```python
from build123d import *

# Parameters (mm, degrees)
SKETCH_R   = 95
SKETCH_R_2 = 7
SKETCH_R_3 = 1.5
SKETCH_R_4 = 2.5
PAD_DEPTH  = 4


with BuildPart() as part:
    # Sketch → Pad (new body)
    with BuildSketch(Plane.XY):
        Circle(SKETCH_R)
        with Locations((-45, 0)):
            Circle(SKETCH_R_2, mode=Mode.SUBTRACT)
        with Locations((45, 0)):
            Circle(SKETCH_R_2, mode=Mode.SUBTRACT)
        with Locations((64.346717, 64.346717)):
            Circle(SKETCH_R_3, mode=Mode.SUBTRACT)
        with Locations((-64.346717, 64.346717)):
            Circle(SKETCH_R_3, mode=Mode.SUBTRACT)
        with Locations((-64.346717, -64.346717)):
            Circle(SKETCH_R_3, mode=Mode.SUBTRACT)
        with Locations((64.346717, -64.346717)):
            Circle(SKETCH_R_3, mode=Mode.SUBTRACT)
        with Locations((-45, 19.5)):
            Circle(SKETCH_R_4, mode=Mode.SUBTRACT)
        with Locations((-28.112505, -9.75)):
            Circle(SKETCH_R_4, mode=Mode.SUBTRACT)
        with Locations((-61.887495, -9.75)):
            Circle(SKETCH_R_4, mode=Mode.SUBTRACT)
        with Locations((45, 19.5)):
            Circle(SKETCH_R_4, mode=Mode.SUBTRACT)
        with Locations((28.112505, -9.75)):
            Circle(SKETCH_R_4, mode=Mode.SUBTRACT)
        with Locations((61.887495, -9.75)):
            Circle(SKETCH_R_4, mode=Mode.SUBTRACT)
        Circle(SKETCH_R_4, mode=Mode.SUBTRACT)
        with Locations((91, 0)):
            Circle(SKETCH_R_3, mode=Mode.SUBTRACT)
        with Locations((-91, 0)):
            Circle(SKETCH_R_3, mode=Mode.SUBTRACT)
        with Locations((0, 91)):
            Circle(SKETCH_R_3, mode=Mode.SUBTRACT)
        with Locations((0, -91)):
            Circle(SKETCH_R_3, mode=Mode.SUBTRACT)
    extrude(amount=PAD_DEPTH)


solid = part.part
```
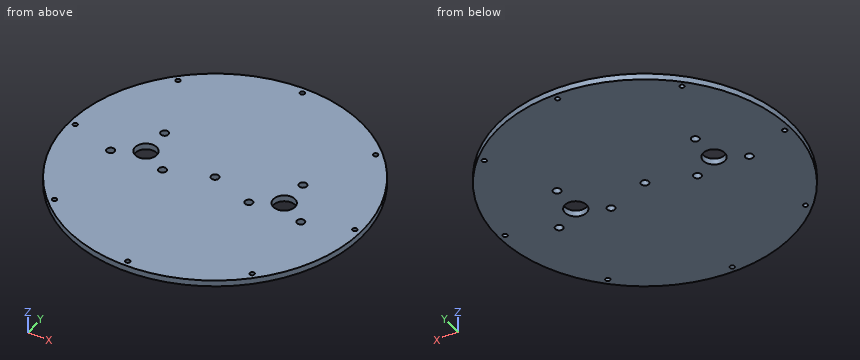
Verification items for the finished model (mm, model axes). Give positions to 0.01 mm unless a question says otherwise; leave off trailing zeros. Order: outer loops, then holes, each group sorted by start corner. A loop starts at its lowest first (then second) coordinate and runs counter-clockwise, first axis right, second up. Notation, with made-up numbers: (87.5, -34) - (111.5, -34) arc R15 ccw to (111.5, -25) - close; hole circle Ø9 at (-23, -8.5). An arc over 180 degrees is marked (long way). Answer as CSV lines item,"result". Start each with the question number.
Item 1: Gauge pin test, flat end, axial feed: pin 1 (1 mm diameter, centred on y = 59.5, z = 1.5, fed in from -X). Record the tip position at first contact, or that the pin passes through.
Item 2: Section check B-B, the plane y = 19.5. Record the boundary of the cut face in (x, z).
Item 3: Material ranges on L1, parallel to Y at x = 0, z = 2.7; L2, parallel to Y at x = -45, z = 1.4; L3, parallel to Y at x = 30, z = 3.3, recorded low to high.
Item 4: Section check D-D, the plane y = -9.75. Record the boundary of the cut face in (x, z), plus the area to 3 significant figures.
Item 5: Section check A-A, the plane x = 45. Record the boundary of the cut face in (y, z).
Item 6: Section check C-C, the plane z = 2.25. State how many separate pieces and enclosed holes the cut face has, plus the area to 3 significant figures.
Filled in:
1,pin 1,"x = -74.46"
2,outline,"(-92.98, 0) - (-47.5, 0) - (-47.5, 4) - (-92.98, 4) - close; (-42.5, 0) - (42.5, 0) - (42.5, 4) - (-42.5, 4) - close; (47.5, 0) - (92.98, 0) - (92.98, 4) - (47.5, 4) - close"
3,L1,"-95 to -92.5, -89.5 to -2.5, 2.5 to 89.5, 92.5 to 95"
3,L2,"-83.67 to -7, 7 to 17, 22 to 83.67"
3,L3,"-90.14 to -11.39, -8.11 to 90.14"
4,outline,"(-94.5, 0) - (-64.39, 0) - (-64.39, 4) - (-94.5, 4) - close; (-59.39, 0) - (-30.61, 0) - (-30.61, 4) - (-59.39, 4) - close; (-25.61, 0) - (25.61, 0) - (25.61, 4) - (-25.61, 4) - close; (30.61, 0) - (59.39, 0) - (59.39, 4) - (30.61, 4) - close; (64.39, 0) - (94.5, 0) - (94.5, 4) - (64.39, 4) - close"
4,area,"676 mm^2"
5,outline,"(-83.67, 0) - (-7, 0) - (-7, 4) - (-83.67, 4) - close; (7, 0) - (17, 0) - (17, 4) - (7, 4) - close; (22, 0) - (83.67, 0) - (83.67, 4) - (22, 4) - close"
6,separate pieces,"1"
6,enclosed holes,"17"
6,area,"27,900 mm^2"
